from build123d import *

# Parameters (mm, degrees)
SKETCH1_R           = 34.8615
SKETCH1_R_2         = 33.274
BOSS_EXTRUDE1_DEPTH = 25.4
SKETCH2_R           = 40.48125
SKETCH2_R_2         = 33.274
BOSS_EXTRUDE2_DEPTH = 4.7625
FILLET1_R           = 5.08
CIRPATTERN1_COUNT   = 6


with BuildPart() as part:
    # Sketch1 → Boss-Extrude1 (new body)
    with BuildSketch(Plane.XY):
        Circle(SKETCH1_R)
        Circle(SKETCH1_R_2, mode=Mode.SUBTRACT)
    extrude(amount=BOSS_EXTRUDE1_DEPTH)

    # Sketch2 → Boss-Extrude2 (add)
    with BuildSketch(Plane.XY.offset(25.4)):
        with Locations(Location((0, 0, 0), (0, 0, 180))):
            Circle(SKETCH2_R)
        Circle(SKETCH2_R_2, mode=Mode.SUBTRACT)
    extrude(amount=BOSS_EXTRUDE2_DEPTH)

    # Fillet1
    fillet1_edges = [part.edges().sort_by_distance(p)[0] for p in [
        (-34.8615, 0, 25.4),
    ]]
    fillet(fillet1_edges, radius=FILLET1_R)

    # Sketch7 → #8-32 Tapped Hole1 (revolve, cut)
    with BuildSketch(Plane(origin=(-18.415, 31.895715621, 30.1625), x_dir=(0, -1, 0), z_dir=(1, 0, 0))):
        Polygon((0, 0), (0, 11.705806461), (1.7272, 10.668), (1.7272, 0), align=None)
    f_8_32_tapped_hole1 = revolve(axis=Axis((-18.415, 31.895715621, 36.5125), (0, 0, -1)), mode=Mode.SUBTRACT)

    # CirPattern1: #8-32 Tapped Hole1 ×6 about axis
    cirpattern1_axis = Axis((0, 0, 0), (0, 0, 1))
    for i in range(1, CIRPATTERN1_COUNT):
        add(f_8_32_tapped_hole1.rotate(cirpattern1_axis, i * 360 / CIRPATTERN1_COUNT), mode=Mode.SUBTRACT)


solid = part.part
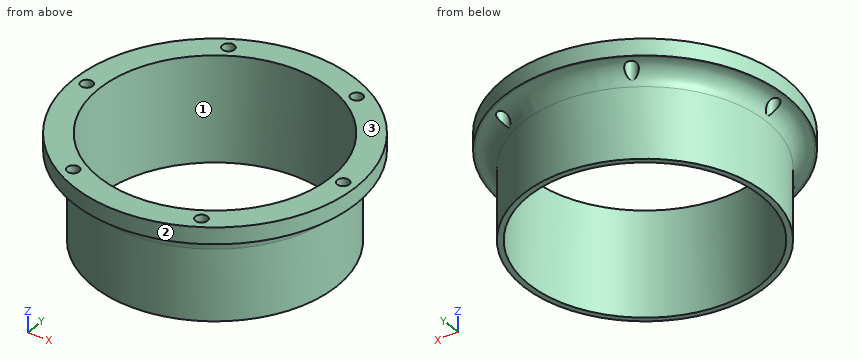
Input: part model. Units: mm. Frame: model coordinates. Face numbers are marked on the shaded views. Round coordinates to 2 decimals unless told otherwise and drop trailing zeros. Loops run counter-clockwise (first coordinate to the right, second up) from the corner with the lowest first, then second, coordinate; pieces in that order, holes last. Notation, with made-up numbers: (-35.75, -30.5) -> (21.25, -30.5) arc R5 ccw to (21.25, -22.5) -> close; hole circle Ø11 at (53.5, 42.25). An arc over 180 degrees is marked (long way). Answer as a JSON object with one key per item and string values. Group by question number.
1) Draft query along Y for the marked faces 1, 2 and 3. Return one class per face: +Y half, -Y half, draft (parallel to the pull), parting line (faces both ways), or undercut.
2) Section query A-A on x = 0. Output: boundary loops of the cut face in (y, z).
3) Section query B-B on z = 10. Output: boundary loops of the cut face in (x, y), plus the area to 3 significant figures.
4) Pin query (flat end, axial travel): pin 1 (8 mm diameter, centred on y = 0, z = 10, fed in from +X); pin 2 (1.5 mm diameter, centred on y = -30, z = 14, fed in from -X); pin 3 (10 mm diameter, centred on x = -10.5, z = 27, fed in from +Y). Return the tip coordinate at first contact, or that it passes through.
5) Ray query, L1, parallel to Y at x = 0, z = 20.5; L2, parallel to Y at x = 28, z = 26; L3, parallel to X at y = 16, z = 5.5. Return the intervals inside material, ascending.
Reply:
{
 "1": {"face 1": "undercut", "face 2": "parting line", "face 3": "draft"},
 "2": {"outline": "(-40.48, 25.4) -> (-39.94, 25.4) arc R5.08 cw to (-34.86, 20.32) -> (-34.86, 0) -> (-33.27, 0) -> (-33.27, 30.16) -> (-40.48, 30.16) -> close; (33.27, 0) -> (34.86, 0) -> (34.86, 20.32) arc R5.08 cw to (39.94, 25.4) -> (40.48, 25.4) -> (40.48, 30.16) -> (33.27, 30.16) -> close"},
 "3": {"outline": "circle Ø69.72 at (0, 0); hole circle Ø66.55 at (0, 0)", "area": "340 mm2"},
 "4": {"pin 1": "stops at x = 34.86", "pin 2": "stops at x = -18.97", "pin 3": "stops at y = 40.11"},
 "5": {"L1": "y = -34.86 to -33.27, 33.27 to 34.86", "L2": "y = -29.24 to -17.98, 17.98 to 29.24", "L3": "x = -30.97 to -29.17, 29.17 to 30.97"}
}
